Here's how the part is built. I have some questions about the finished solid (model axes, mm). A direction names the side the tool comes from. Coordinates: 2 decimals unless noted, no trailing zeros. Loops run counter-clockwise (first coordinate to the right, second up) from the corner with the lowest first, then second, coordinate; pieces in that order, holes last. Notation, with made-up numbers: M -17.5,-18.5 L -5.5,-18.5 A13 ccw -5.5,-9.5 Z; hole C 40,-9 d8. An arc over 180 degrees is marked long. Use CSV: the item, a comma, the result in double quotes. Start each with the question number.
Q1. Which directions (+Z, -Z, +X, -X, +Y, -Y) give clear straight access to the entire face, cutting with the end or side of a thin tool? Please do faces 1 (the flat face through (0, 0, -1)), 2 (the flat face through (0, 13, 11.989)).
Q2. If we mould it in two halves opening along X, with no side actions, what happens to faces 3 (the cylindrical face through (9.54, 26.61, -12.69)), 4 (the flat face through (0, 53.975, -1)), 5 (the flat face through (-6.35, 27, 13))? For each: +X half, -X half, draft (parallel to the pull), parting line (faces both ways), or undercut.
Q3. If we section it at A-A (x = 0): Please give me the cut outline in (y, z) (3 decimals).
Q4. If we section it at C-C (y = 41): Please give me the cut outline in (x, z) (3 decimals), and give its area (3 significant figures).
Q5. For pin 1 Ø5 at (x, y) = (-7.5, 12.5) entering from -Z; pin 2 Ø10 at (x, y) = (1, 46) entering from +Z; pin 3 Ø10 at (x, y) = (0, 31.75) entering from +Z; pin 4 Ø3 at (y, z) = (23.5, 13) entering from -X, each with a flat end and sliding along its axis, tell me the tip position at first contact or that it passes through.
Q6. Please list where these lines run through material, in increasing order: probe 1 along Y at (x, z) = (0, 2) (3 decimals); probe 2 along X at (y, z) = (36, -6.5); probe 3 along X at (y, z) = (31.75, 4). Write a range as [from, to].
Q7. If we section it at D-D (z = -4): Please give me the cut outline in (x, y) (3 decimals), and give its area (3 significant figures).
Q8. If we section it at B-B (z = 0): Please give me the cut outline in (x, y) (3 decimals), and give its area (3 significant figures).
from build123d import *

# Parameters (mm, degrees)
SKETCH1_R           = 15.875
CYLINDER_DEPTH      = 53.975
SKETCH2_W           = 12.7
SKETCH2_H           = 3.8862
FLUE_TRACK_DEPTH    = 76.2
AIR_DUCT_DEPTH      = 59.45794963
AIR_DUCT_DEPTH_BACK = 59.45794963
SKETCH3_R           = 6.35


with BuildPart() as part:
    # Sketch1 → cylinder (new body)
    with BuildSketch(Plane(origin=(0, 0, 0), x_dir=(1, 0, 0), z_dir=(0, 1, 0))):
        with Locations(Location((0, 0, 0), (0, 0, 270))):
            Circle(SKETCH1_R)
    extrude(amount=CYLINDER_DEPTH)

    # Sketch2 → flue track (cut)
    with BuildSketch(Plane(origin=(0, 53.975, 0), x_dir=(1, 0, 0), z_dir=(0, 1, 0))):
        with Locations((0, -13.9319)):
            Rectangle(SKETCH2_W, SKETCH2_H)
    extrude(amount=-FLUE_TRACK_DEPTH, mode=Mode.SUBTRACT)

    # Sketch3 → air duct (cut, two sides: drawn at the far end of the back side and taken through both)
    with BuildSketch(Plane.XY.offset(-AIR_DUCT_DEPTH_BACK)):
        with Locations((0, 31.75)):
            Circle(SKETCH3_R)
    extrude(amount=AIR_DUCT_DEPTH + AIR_DUCT_DEPTH_BACK, mode=Mode.SUBTRACT)


solid = part.part
Results below:
1,face 1,"+Z, -Z, +X, -X, -Y"
1,face 2,"+Z, +Y, -Y"
2,face 3,"parting line"
2,face 4,"draft"
2,face 5,"undercut"
3,outline,"M 0,-15.875 L 25.4,-15.875 L 25.4,11.989 L 0,11.989 Z; M 38.1,-15.875 L 53.975,-15.875 L 53.975,11.989 L 38.1,11.989 Z"
4,outline,"M -6.35,11.989 L -6.35,14.55 A15.875 ccw long 6.35,14.55 L 6.35,11.989 Z"
4,area,"748 mm^2"
5,pin 1,"z = -15.07"
5,pin 2,"z = 11.99"
5,pin 3,"through"
5,pin 4,"x = -10.94"
6,probe 1,"[0, 25.4], [38.1, 53.975]"
6,probe 2,"[-14.48, -4.72], [4.72, 14.48]"
6,probe 3,"[-15.36, -6.35], [6.35, 15.36]"
7,outline,"M -15.363,0 L 15.363,0 L 15.363,53.975 L -15.363,53.975 Z; hole C 0,31.75 d12.7"
7,area,"1,530 mm^2"
8,outline,"M -15.875,0 L 15.875,0 L 15.875,53.975 L -15.875,53.975 Z; hole C 0,31.75 d12.7"
8,area,"1,590 mm^2"
